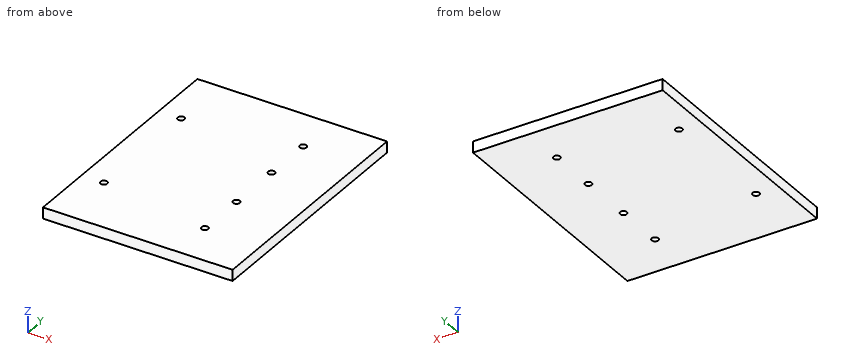
```python
from build123d import *

# Parameters (mm, degrees)
SKETCH1_W           = 170
SKETCH1_H           = 110
BOSS_EXTRUDE1_DEPTH = 5
SKETCH2_R           = 1.5
CUT_EXTRUDE1_DEPTH  = 6
SKETCH3_R           = 1.5
CUT_EXTRUDE2_DEPTH  = 6
SKETCH4_W           = 40.789310726
SKETCH4_H           = 120.699967799
CUT_EXTRUDE3_DEPTH  = 86


with BuildPart() as part:
    # Sketch1 → Boss-Extrude1 (new body)
    with BuildSketch(Plane.XY):
        Rectangle(SKETCH1_W, SKETCH1_H)
    extrude(amount=BOSS_EXTRUDE1_DEPTH)

    # Sketch2 → Cut-Extrude1 (cut, through all)
    with BuildSketch(Plane.XY.offset(5)):
        with Locations((-75, 27.5)):
            Circle(SKETCH2_R)
        with Locations((-75, -27.5)):
            Circle(SKETCH2_R)
        with Locations((75, -27.5)):
            Circle(SKETCH2_R)
        with Locations((75, 27.5)):
            Circle(SKETCH2_R)
    extrude(amount=-CUT_EXTRUDE1_DEPTH, mode=Mode.SUBTRACT)

    # Sketch3 → Cut-Extrude2 (cut, through all)
    with BuildSketch(Plane.XY.offset(5)):
        with Locations((-25, 35)):
            Circle(SKETCH3_R)
        with Locations((-25, 12.5)):
            Circle(SKETCH3_R)
        with Locations((-25, -12.5)):
            Circle(SKETCH3_R)
        with Locations((-25, -35)):
            Circle(SKETCH3_R)
        with Locations((25, -35)):
            Circle(SKETCH3_R)
        with Locations((25, -12.5)):
            Circle(SKETCH3_R)
        with Locations((25, 12.5)):
            Circle(SKETCH3_R)
        with Locations((25, 35)):
            Circle(SKETCH3_R)
    extrude(amount=-CUT_EXTRUDE2_DEPTH, mode=Mode.SUBTRACT)

    # Sketch4 → Cut-Extrude3 (cut, through all)
    with BuildSketch(Plane(origin=(0, 0, 0), x_dir=(0, 0, -1), z_dir=(1, 0, 0))):
        with Locations((-5.456845945, -1.288881565)):
            Rectangle(SKETCH4_W, SKETCH4_H)
    extrude(amount=CUT_EXTRUDE3_DEPTH, mode=Mode.SUBTRACT)


solid = part.part
```
Geometry check sheet. Reference: the model listing, model coordinates, mm. Coordinates: 2 decimals unless noted, no trailing zeros. Order: outer loops, then holes, each group sorted by start corner. A loop starts at its lowest first (then second) coordinate and runs counter-clockwise, first axis right, second up.
Q1. Thickness scan on probe 1 along Y at (x, z) = (-25, 1.6); probe 2 along X at (y, z) = (35.5, 1.2). Record the ranges inside material, lowest first.
Reply:
probe 1: y = -55 to -36.5, -33.5 to -14, -11 to 11, 14 to 33.5, 36.5 to 55
probe 2: x = -85 to -26.41, -23.59 to 0
Q2. Sectioned sample at A-A on y = 27.5. Record the cut outline in (x, z).
Reply:
outline: (-85, 0) - (-76.5, 0) - (-76.5, 5) - (-85, 5) - close; (-73.5, 0) - (0, 0) - (0, 5) - (-73.5, 5) - close
Q3. Sectioned sample at C-C on x = -25. Record the cut outline in (y, z).
Reply:
outline: (-55, 0) - (-36.5, 0) - (-36.5, 5) - (-55, 5) - close; (-33.5, 0) - (-14, 0) - (-14, 5) - (-33.5, 5) - close; (-11, 0) - (11, 0) - (11, 5) - (-11, 5) - close; (14, 0) - (33.5, 0) - (33.5, 5) - (14, 5) - close; (36.5, 0) - (55, 0) - (55, 5) - (36.5, 5) - close
Q4. Sectioned sample at B-B on x = -75. Record the cut outline in (y, z), and give its area (3 significant figures).
Reply:
outline: (-55, 0) - (-29, 0) - (-29, 5) - (-55, 5) - close; (-26, 0) - (26, 0) - (26, 5) - (-26, 5) - close; (29, 0) - (55, 0) - (55, 5) - (29, 5) - close
area: 520 mm2
